Here's how the part is built. I have some questions about the finished solid (model axes, mm). A direction names the side the tool comes from. Coordinates: 2 decimals unless noted, no trailing zeros. Loops run counter-clockwise (first coordinate to the right, second up) from the corner with the lowest first, then second, coordinate; pieces in that order, holes last.
from build123d import *

# Parameters (mm, degrees)
F0_R     = 3.25
F0_R_2   = 1
F1_DEPTH = 11.5
F0_R_3   = 4.25
F2_DEPTH = 4
F3_R     = 0.2
F4_R     = 0.5


with BuildPart() as f1:
    # F0 (on Top) → F1 (new body)
    with BuildSketch(Plane.XY):
        Circle(F0_R)
        Circle(F0_R_2, mode=Mode.SUBTRACT)
    extrude(amount=F1_DEPTH)

    # F0 (on Top) → F2 (join)
    with BuildSketch(Plane.XY):
        Circle(F0_R_3)
        Circle(F0_R, mode=Mode.SUBTRACT)
    extrude(amount=F2_DEPTH)

    # F3
    f3_edges = [f1.edges().sort_by_distance(p)[0] for p in [
        (-1, 0, 11.5),
    ]]
    fillet(f3_edges, radius=F3_R)

    # F4
    f4_edges = [f1.edges().sort_by_distance(p)[0] for p in [
        (-1, 0, 0),
    ]]
    fillet(f4_edges, radius=F4_R)


solid = f1.part
Q1. Suppose I cut it at A-A on x = 0. Write out the boundary of the cut face in (y, z).
Q2. Will these pins go through, and if not, where does the flat tip stop? P1, Ø5, axis at y = -3, z = 8.5, coming from the +X side; P2, Ø5, axis at x = -0.5, z = 9, coming from the +Y side; P3, Ø4, axis at x = -3, z = 8, coming from the +Y side.
Q3. Suppose I cut it at D-D on x = 2.5. Write out the boundary of the cut face in (y, z).
Q4. We'd pull the mould along Y, two halves only. Please class faces 1 (the cylindrical face through (0, -1, 6)), 2 (the cylindrical face through (2.285, 3.584, 1.972)), 3 (the flat face through (2, 0, 0)): pulls with the +Y half, pulls with the -Y half, needs draft (parallel to the pull), parting line crosses it, or undercut.
Q5. For faces 4 (the cylindrical face through (-2.579, -1.978, 7.698)), 5 (the flat face through (1.4, 0, 11.5)), which set-ups out of +Z, -Z, +X, -X, +Y, -Y let a thin tool reach every point of the face, with its end or its side?
Q6. Suppose I cut it at C-C on z = 4.25. Write out the boundary of the cut face in (x, y), and give its area (3 significant figures).
Q7. Please list where these lines run through material, in increasing order: probe 1 along Y at (x, z) = (0, 6); probe 2 along Y at (x, z) = (0, 3.5); probe 3 along X at (y, z) = (-0.5, 2.5).
Check values:
1. outline: (-4.25, 0) - (-1.5, 0) arc R0.5 ccw to (-1, 0.5) - (-1, 11.3) arc R0.2 ccw to (-1.2, 11.5) - (-3.25, 11.5) - (-3.25, 4) - (-4.25, 4) - close; (1, 0.5) arc R0.5 ccw to (1.5, 0) - (4.25, 0) - (4.25, 4) - (3.25, 4) - (3.25, 11.5) - (1.2, 11.5) arc R0.2 ccw to (1, 11.3) - close
2. P1: stops at x = 3.21
2. P2: stops at y = 3.25
2. P3: stops at y = 3.09
3. outline: (-3.44, 0) - (3.44, 0) - (3.44, 4) - (2.08, 4) - (2.08, 11.5) - (-2.08, 11.5) - (-2.08, 4) - (-3.44, 4) - close
4. face 1: undercut
4. face 2: parting line crosses it
4. face 3: needs draft
5. face 4: +Z
5. face 5: +Z, +X, -X, +Y, -Y
6. outline: circle Ø6.5 at (0, 0); hole circle Ø2 at (0, 0)
6. area: 30.0 mm2
7. probe 1: y = -3.25 to -1, 1 to 3.25
7. probe 2: y = -4.25 to -1, 1 to 4.25
7. probe 3: x = -4.22 to -0.87, 0.87 to 4.22
